Part model, mm, in its own coordinate system. Face numbers are marked on the shaded views. A direction names the side the tool comes from. Round coordinates to 2 decimals unless told otherwise and drop trailing zeros. Loops run counter-clockwise (first coordinate to the right, second up) from the corner with the lowest first, then second, coordinate; pieces in that order, holes last.
(1) Cut at A-A on y = -40. List the corners of the cut face in (x, z).
(2) Mould opens along Y. For the marked faces 1, 2 and 3 say: +Y half, -Y half, draft (parallel to the pull), parting line (faces both ways), or undercut.
(3) Cut at C-C on x = -18. List the corners of the cut face in (y, z).
(4) Tool access for the marked faces 4, 5, 6 and 7: list every direction of +Z, -Z, +X, -X, +Y, -Y with a clear straight run to the whole face (end or side of a thin tool).
(5) Cut at D-D on z = 46. List the corners of the cut face in (x, y).
(6) Probe probe 1 along Y at (x, z) = (-22.5, 37); probe 2 along X at (y, z) = (-31.5, 22); probe 3 along Y at (x, z) = (80, 41). List the from-to ranges inside material, lowest first.
(7) Flat gauge pins, fed straight in: pin 1 (10 mm diameter, centred on y = -3.5, z = 68, fed in from -X); pin 2 (8 mm diameter, centred on x = 31.5, y = -75, fed in from +Z); pin 3 (22 mm diameter, centred on x = 118, z = 71, fed in from +Y). Where does each tip first touch, or does it go through?
(8) Cut at B-B on z = 63.5. List the corners of the cut face in (x, y).
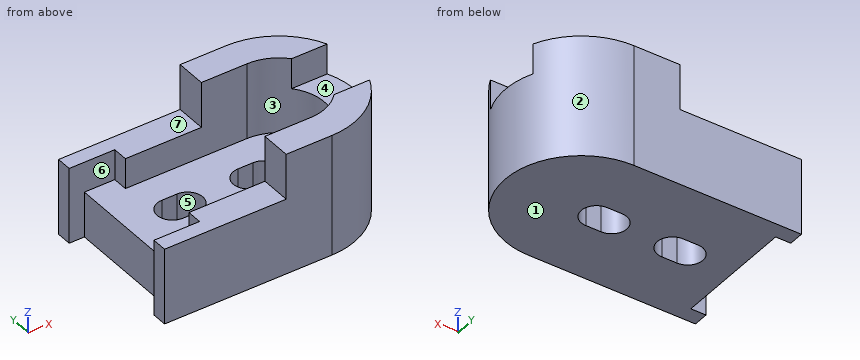
from build123d import *

# Parameters (mm, degrees)
BOSS_EXTRUDE1_DEPTH      = 50
BOSS_EXTRUDE2_DEPTH      = 30
BOSS_EXTRUDE3_DEPTH      = 50
BOSS_EXTRUDE7_DEPTH      = 50
BOSS_EXTRUDE7_DEPTH_BACK = 30
SKETCH5_W                = 20
SKETCH5_H                = 40
CUT_EXTRUDE1_DEPTH       = 211
CUT_EXTRUDE2_DEPTH       = 211
CUT_EXTRUDE3_DEPTH       = 211


with BuildPart() as part:
    # Sketch1 → Boss-Extrude1 (new body)
    with BuildSketch(Plane.XY):
        Polygon((0, 0), (-30, 0), (-30, 10), (50, 10), (50, -10), (0, -10), align=None)
    extrude(amount=BOSS_EXTRUDE1_DEPTH)

    # Sketch2 → Boss-Extrude2 (add)
    with BuildSketch(Plane(origin=(0, 0, 0), x_dir=(-1, 0, 0), z_dir=(0, 0, -1))):
        with BuildLine():
            Line((0, 0), (0, -10))
            Line((0, -10), (-50, -10))
            Line((-50, -10), (-80, -10))
            ThreePointArc((-80, -10), (-110, -40), (-80, -70))
            Line((-80, -70), (0, -70))
            Line((0, -70), (0, -80))
            Line((0, -80), (20, -80))
            Line((20, -80), (20, 0))
            Line((20, 0), (0, 0))
        make_face()
    extrude(amount=-BOSS_EXTRUDE2_DEPTH)

    # Sketch3 → Boss-Extrude3 (add)
    with BuildSketch(Plane(origin=(0, 0, 0), x_dir=(-1, 0, 0), z_dir=(0, 0, -1))):
        Polygon((0, -70), (0, -80), (30, -80), (30, -90), (-50, -90), (-50, -70), align=None)
    extrude(amount=-BOSS_EXTRUDE3_DEPTH)

    # Sketch4 → Boss-Extrude7 (add, two sides)
    with BuildSketch(Plane.XY.offset(30)) as boss_extrude7_sk:
        with BuildLine():
            Line((80, -90), (50, -90))
            Line((50, -90), (50, -70))
            Line((50, -70), (80, -70))
            ThreePointArc((80, -70), (110, -40), (80, -10))
            Line((80, -10), (50, -10))
            Line((50, -10), (50, 10))
            Line((50, 10), (80, 10))
            ThreePointArc((80, 10), (130, -40), (80, -90))
        make_face()
    extrude(amount=BOSS_EXTRUDE7_DEPTH)
    extrude(boss_extrude7_sk.sketch, amount=-BOSS_EXTRUDE7_DEPTH_BACK)

    # Sketch5 → Cut-Extrude1 (cut)
    with BuildSketch(Plane(origin=(0, 0, 0), x_dir=(0, 0, -1), z_dir=(1, 0, 0))):
        with Locations((-70, -40)):
            Rectangle(SKETCH5_W, SKETCH5_H)
    extrude(amount=CUT_EXTRUDE1_DEPTH, mode=Mode.SUBTRACT)

    # Sketch6 → Cut-Extrude2 (cut)
    with BuildSketch(Plane.XY.offset(30)):
        with BuildLine():
            Line((10, -30), (20, -30))
            ThreePointArc((20, -30), (30, -40), (20, -50))
            Line((20, -50), (10, -50))
            ThreePointArc((10, -50), (0, -40), (10, -30))
        make_face()
    extrude(amount=-CUT_EXTRUDE2_DEPTH, mode=Mode.SUBTRACT)

    # Sketch7 → Cut-Extrude3 (cut)
    with BuildSketch(Plane.XY.offset(30)):
        with BuildLine():
            Line((70, -30), (60, -30))
            ThreePointArc((60, -30), (50, -40), (60, -50))
            Line((60, -50), (70, -50))
            ThreePointArc((70, -50), (80, -40), (70, -30))
        make_face()
    extrude(amount=-CUT_EXTRUDE3_DEPTH, mode=Mode.SUBTRACT)


solid = part.part
Final values:
1. outline: (-20, 0) - (0, 0) - (0, 30) - (-20, 30) - close; (30, 0) - (50, 0) - (50, 30) - (30, 30) - close; (80, 0) - (130, 0) - (130, 60) - (110, 60) - (110, 30) - (80, 30) - close
2. face 1: draft
2. face 2: parting line
2. face 3: undercut
3. outline: (-90, 0) - (10, 0) - (10, 50) - (0, 50) - (0, 30) - (-80, 30) - (-80, 50) - (-90, 50) - close
4. face 4: +Z, +X, -X
4. face 5: +Z, -Z
4. face 6: +Z, -X
4. face 7: +Z, -X, +Y, -Y
5. outline: (-30, -90) - (80, -90) arc R50 ccw to (80, 10) - (-30, 10) - (-30, 0) - (0, 0) - (0, -10) - (80, -10) arc R30 cw to (80, -70) - (0, -70) - (0, -80) - (-30, -80) - close
6. probe 1: y = -90 to -80, 0 to 10
6. probe 2: x = -20 to 4.73, 25.27 to 54.73, 75.27 to 129.27
6. probe 3: y = -90 to -70, -10 to 10
7. pin 1: stops at x = 50
7. pin 2: stops at z = 50
7. pin 3: stops at y = 2.08
8. outline: (50, -90) - (80, -90) arc R50 ccw to (125.83, -60) - (102.36, -60) arc R30 cw to (80, -70) - (50, -70) - close; (50, -10) - (80, -10) arc R30 cw to (102.36, -20) - (125.83, -20) arc R50 ccw to (80, 10) - (50, 10) - close
